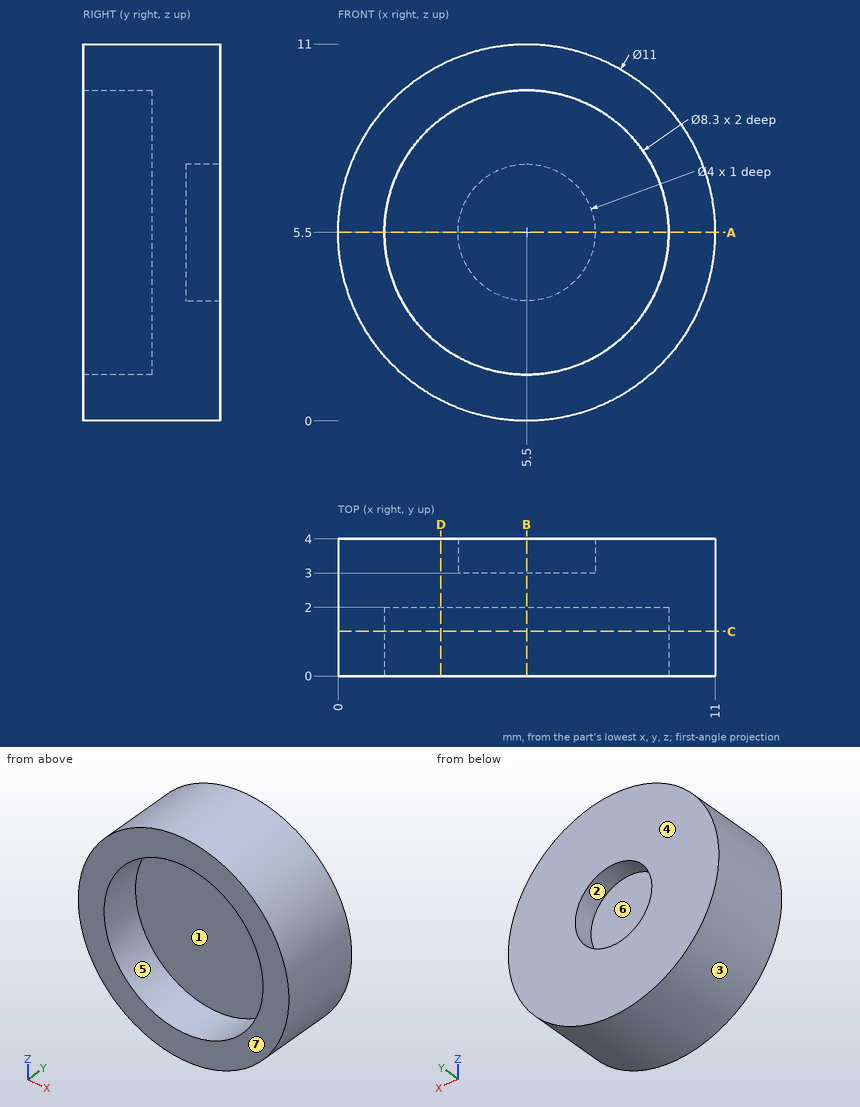
Geometry: see drawing. Coordinates: mm, zero at the bounding-box minimum. A direction names the side the tool comes from. Round coordinates to 2 decimals unless told otherwise and drop trailing zeros. Write each loop counter-clockwise with the first axis right and the second up, starting at its lowest first coordinate (ties: lowest second). Pieces come first, ordered by that corner, then holes.
1) Cut plane C-C (y = 1.3). Return the cut outline in (x, z), then the cut area to 3 significant figures.
2) Cut plane B-B (x = 5.5). Return the cut outline in (y, z), then the cut area to 3 significant figures.
3) Reachability of the marked faces 5, 6 and 7 from +Z, -Z, +X, -X, +Y, -Y: full face, straight path, thin tool, end or side. Return the list, or none.
4) Contact query for flat-ended pins moving along their axis: P1, Ø5, axis at x = 5.5, z = 5.5, coming from the -Y side; P2, Ø2, axis at x = 3, y = 0.5, coming from the +Z side. Output: stop coordinate, or through.
5) Draft query along X for the marked faces 1, 2, 3 and 4. Return one class per face: pulls with the +X half, pulls with the -X half, needs draft (parallel to the pull), parting line crosses it, or undercut.
6) Cut plane A-A (z = 5.5). Return the cut outline in (x, y).
7) Ray query, L1, parallel to X at y = 3.4, z = 5.5; L2, parallel to X at y = 1.35, z = 6; L3, parallel to Y at x = 2.75, z = 4. Return the intervals inside material, ascending.
8) Cut plane D-D (x = 3). Return the cut outline in (y, z), then the cut area to 3 significant figures.
Geometry says:
1. outline: circle Ø11 at (5.5, 5.5); hole circle Ø8.3 at (5.5, 5.5)
1. area: 40.9 mm2
2. outline: (0, 0) - (4, 0) - (4, 3.5) - (3, 3.5) - (3, 7.5) - (4, 7.5) - (4, 11) - (0, 11) - (0, 9.65) - (2, 9.65) - (2, 1.35) - (0, 1.35) - close
2. area: 23.4 mm2
3. face 5: -Y
3. face 6: +Y
3. face 7: +Z, -Z, +X, -X, -Y
4. P1: stops at y = 2
4. P2: stops at z = 10.79
5. face 1: undercut
5. face 2: undercut
5. face 3: parting line crosses it
5. face 4: needs draft
6. outline: (0, 0) - (1.35, 0) - (1.35, 2) - (9.65, 2) - (9.65, 0) - (11, 0) - (11, 4) - (7.5, 4) - (7.5, 3) - (3.5, 3) - (3.5, 4) - (0, 4) - close
7. L1: x = 0 to 3.5, 7.5 to 11
7. L2: x = 0.02 to 1.38, 9.62 to 10.98
7. L3: y = 2 to 4
8. outline: (0, 0.6) - (4, 0.6) - (4, 10.4) - (0, 10.4) - (0, 8.81) - (2, 8.81) - (2, 2.19) - (0, 2.19) - close
8. area: 25.9 mm2
